Autodesk Inventor part; units mm, degrees
ref_plane "YZ Plane" through (0, 0, 0) normal (1, 0, 0) x (0, 1, 0)
ref_plane "XZ Plane" through (0, 0, 0) normal (0, 1, 0) x (-1, 0, 0)
ref_plane "XY Plane" through (0, 0, 0) normal (0, 0, 1) x (1, 0, 0)
sketch "Sketch1" plane through (0, 0, 0) normal (0, 0, 1) x (1, 0, 0)
  line L0 (0, 0) -> (2.5, 0)
  line L1 (2.5, 0) -> (2.5, -5)
  line L2 (2.5, -5) -> (22.5, -5)
  line L3 (22.5, -5) -> (22.5, 0)
  line L4 (22.5, 0) -> (25, 0)
  line L5 (25, 0) -> (25, 15)
  line L6 (25, 15) -> (22.5, 15)
  line L7 (22.5, 15) -> (22.5, 20)
  line L8 (22.5, 20) -> (2.5, 20)
  line L9 (2.5, 20) -> (2.5, 15)
  line L10 (2.5, 15) -> (0, 15)
  line L11 (0, 15) -> (0, 0)
  circle A0 centre (12.5, 7.5) radius 1.6
  point P0 (0, 7.5)
  point P1 (12.5, 20)
  dimension "d0" = 20
  dimension "d1" = 15
  dimension "d2" = 25
  dimension "d3" = 5
  dimension "d4" = 3.2
extrude "Extrusion1" add sketch "Sketch1" along normal blind 6.731
equation "\"d10\" = THICKB"
equation "\"THICKA\" = 3.175"
equation "\"THICKB\" = 6.731"
equation "\"THICKC\" = 12.7"
equation "\"BALLDIA\" = 12"
equation "\"MAGDIA\" = 9.5"
equation "\"THICKPLY\" = 5"
properties part number "Frame_Upper_Plate_Pulley_A"
Can you work these out from the model? Positions are in its coordinate system, mm. A direction names the side the tool comes from. Coordinates: 2 decimals unless noted, no trailing zeros. Loops run counter-clockwise (first coordinate to the right, second up) from the corner with the lowest first, then second, coordinate; pieces in that order, holes last. Notation, with made-up numbers: (-16.75, 5) -> (-2.75, 5) arc R17 ccw to (-2.75, 22) -> close; hole circle Ø5 at (71, 55). An arc over 180 degrees is marked (long way). Put each result on its own line as item: value. Start each with the question number.
Q1. For faces 1 (the face through (2.5, 18, 3)), 2 (the face through (10, 8, 6.731)), 3 (the face through (22.5, 17, 3)), 4 (the face through (2.5, -2, 3)), 5 (the face through (22.5, -3, 3)), which set-ups out of +Z, -Z, +X, -X, +Y, -Y let a thin tool reach every point of the face, with its end or its side?
Q2. I'm going to push flat-ended pins straight in: P1, Ø2, axis at x = 1, z = 2.5, coming from the +Y side; P2, Ø2.5, axis at y = 16.5, z = 2.5, coming from the -X side; P3, Ø3, axis at x = 12.5, y = 7.5, coming from the -Z side; P4, Ø0.8, axis at x = 1.5, z = 4.5, coming from the -Y side. Where does each tip first touch, or does it pass through?
Q3. I want a section at A-A (x = 12.5). Write out the boundary of the cut face in (y, z).
Q4. I want a section at C-C (y = 7.5). Write out the boundary of the cut face in (x, z), plus the area to 3 significant figures.
Q5. Thinking about a two-plate mould opening in Y: for faces 6 (the face through (25, 7, 3)), 7 (the face through (11.23, 8.47, 3.32)), 8 (the face through (12, -5, 3)), which applies, pulls with the +Y half, pulls with the -Y half, needs draft (parallel to the pull), parting line crosses it, or undercut?
Q6. I want a section at D-D (y = -2.75). Write out the boundary of the cut face in (x, z), plus the area to 3 significant figures.
Q7. I want a section at B-B (z = 4.5). Write out the boundary of the cut face in (x, y), plus the area to 3 significant figures.
Q8. If I drill on line 1 (Y direction, x = 12.5, z = 4.25); line 2 (Y direction, x = 1.5, z = 4); line 3 (X direction, y = 6.25, z = 3.5), over which ranges is the centre line in solid material (lowest first)? Write a range as [from, to].
Taken from the geometry:
1. face 1: +Z, -Z, -X, +Y
1. face 2: +Z, +X, -X, +Y, -Y
1. face 3: +Z, -Z, +X, +Y
1. face 4: +Z, -Z, -X, -Y
1. face 5: +Z, -Z, +X, -Y
2. P1: stops at y = 15
2. P2: stops at x = 2.5
2. P3: passes through
2. P4: stops at y = 0
3. outline: (-5, 0) -> (5.9, 0) -> (5.9, 6.73) -> (-5, 6.73) -> close; (9.1, 0) -> (20, 0) -> (20, 6.73) -> (9.1, 6.73) -> close
4. outline: (0, 0) -> (10.9, 0) -> (10.9, 6.73) -> (0, 6.73) -> close; (14.1, 0) -> (25, 0) -> (25, 6.73) -> (14.1, 6.73) -> close
4. area: 147 mm2
5. face 6: needs draft
5. face 7: undercut
5. face 8: pulls with the -Y half
6. outline: (2.5, 0) -> (22.5, 0) -> (22.5, 6.73) -> (2.5, 6.73) -> close
6. area: 135 mm2
7. outline: (0, 0) -> (2.5, 0) -> (2.5, -5) -> (22.5, -5) -> (22.5, 0) -> (25, 0) -> (25, 15) -> (22.5, 15) -> (22.5, 20) -> (2.5, 20) -> (2.5, 15) -> (0, 15) -> close; hole circle Ø3.2 at (12.5, 7.5)
7. area: 567 mm2
8. line 1: y = [-5, 5.9], [9.1, 20]
8. line 2: y = [0, 15]
8. line 3: x = [0, 11.5], [13.5, 25]
